Part model, mm, in its own coordinate system. Round coordinates to 2 decimals unless told otherwise and drop trailing zeros. Loops run counter-clockwise (first coordinate to the right, second up) from the corner with the lowest first, then second, coordinate; pieces in that order, holes last. Notation, with made-up numbers: (-33, -18) -> (-12, -18) arc R31 ccw to (-12, 11) -> close; hole circle Ø1 at (70, -15.75). An arc over 180 degrees is marked (long way). Answer as CSV lines item,"result".
from build123d import *

# Parameters (mm, degrees)
ESBO_O3_R                = 4
RESSALTO_EXTRUS_O1_DEPTH = 183.5
CHANFRO1_SIZE            = 0.5


with BuildPart() as part:
    # Esboço3 → Ressalto-extrusão1 (new, symmetric)
    with BuildSketch(Plane(origin=(0, 0, 0), x_dir=(1, 0, 0), z_dir=(0, 1, 0))):
        with Locations(Location((0, 0, 0), (0, 0, 270))):
            Circle(ESBO_O3_R)
    extrude(amount=RESSALTO_EXTRUS_O1_DEPTH, both=True)

    # Chanfro1
    chanfro1_edges = [part.edges().sort_by_distance(p)[0] for p in [
        (0, -183.5, -4),
        (0, 183.5, -4),
    ]]
    chamfer(chanfro1_edges, length=CHANFRO1_SIZE)

    # Esboço4 → Furo roscado de M51 (revolve, cut)
    with BuildSketch(Plane(origin=(0, 183.5, 0), x_dir=(0, 0, 1), z_dir=(1, 0, 0))):
        Polygon((0, 0), (0, 25.2618073), (2.1, 24), (2.1, 0), align=None)
    furo_roscado_de_m51 = revolve(axis=Axis((0, 189.85, 0), (0, -1, 0)), mode=Mode.SUBTRACT)

    # Espelhar1: Furo roscado de M51 across plane
    add(furo_roscado_de_m51.mirror(Plane.ZX), mode=Mode.SUBTRACT)


solid = part.part
Q1. Drill centre lines: line 1 along X through (y, z) = (178.25, 0); line 2 along X through (y, z) = (88, -2). Where is each one in solid material? Low to high.
Geometry results:
line 1,"-4 to -2.1, 2.1 to 4"
line 2,"-3.46 to 3.46"
Q2. Saw through at A-A, the plane y = -22. Write the cut outline in (x, z), then the cut area to 3 significant figures.
Geometry results:
outline,"circle Ø8 at (0, 0)"
area,"50.3 mm2"
Q3. Drop flat-ended pins along their axis: P1, Ø4, axis at y = -81, z = -2, coming from the -X side; P2, Ø1, axis at x = -1.5, y = -30.5, coming from the +Z side; P3, Ø1.5, axis at x = -1.5, y = 130, coming from the -Z side. Give the stop position or say it passes through.
Geometry results:
P1,"x = -4"
P2,"z = 3.87"
P3,"z = -3.93"
